from build123d import *

# Parameters (mm, degrees)
SKETCH1_W           = 164.45
SKETCH1_H           = 80
SKETCH1_R           = 2.5
SKETCH1_W_2         = 43.25
SKETCH1_H_2         = 50
BOSS_EXTRUDE1_DEPTH = 3.1
SKETCH2_W           = 3.1
SKETCH2_H           = 39.596362368
SKETCH2_H_2         = 40
CUT_EXTRUDE1_DEPTH  = 4.1
FILLET1_R           = 25
SKETCH3_R           = 2.5
BOSS_EXTRUDE2_DEPTH = 3.1
FILLET3_R           = 10
FILLET4_R           = 20


with BuildPart() as part:
    # Sketch1 → Boss-Extrude1 (new body)
    with BuildSketch(Plane.XY):
        Rectangle(SKETCH1_W, SKETCH1_H)
        Circle(SKETCH1_R, mode=Mode.SUBTRACT)
        with BuildLine():
            Line((-76.75, -15.97), (-76.75, 15.97))
            ThreePointArc((-76.75, 15.97), (-75, 17.72), (-73.25, 15.97))
            Line((-73.25, 15.97), (-73.25, -15.97))
            ThreePointArc((-73.25, -15.97), (-75, -17.72), (-76.75, -15.97))
        make_face(mode=Mode.SUBTRACT)
        with BuildLine():
            Line((18.725, -15.97), (18.725, 15.97))
            ThreePointArc((18.725, 15.97), (20.475, 17.72), (22.225, 15.97))
            Line((22.225, 15.97), (22.225, -15.97))
            ThreePointArc((22.225, -15.97), (20.475, -17.72), (18.725, -15.97))
        make_face(mode=Mode.SUBTRACT)
        with Locations((-36.625, 0)):
            Rectangle(SKETCH1_W_2, SKETCH1_H_2, mode=Mode.SUBTRACT)
    extrude(amount=BOSS_EXTRUDE1_DEPTH)

    # Sketch2 → Cut-Extrude1 (cut, through all)
    with BuildSketch(Plane.XY.offset(3.1)):
        with Locations((61.575, -20.201818816)):
            Rectangle(SKETCH2_W, SKETCH2_H)
        with Locations((80.675, -20)):
            Rectangle(SKETCH2_W, SKETCH2_H_2)
    extrude(amount=-CUT_EXTRUDE1_DEPTH, mode=Mode.SUBTRACT)

    # Fillet1
    fillet1_edges = [part.edges().sort_by_distance(p)[0] for p in [
        (-82.225, -40, 1.55),
        (-82.225, 40, 1.55),
    ]]
    fillet(fillet1_edges, radius=FILLET1_R)

    # Sketch3 → Boss-Extrude2 (add)
    with BuildSketch(Plane.XY.offset(3.1)):
        with BuildLine():
            add(Edge.make_bspline(
                [(82.225, 40), (100.790922155, 40.44036534), (122.998075296, 29.670027282), (145.632337886, 10.163727788), (160, 10)],
                knots=[0, 0, 0, 0, 0.531248583, 1, 1, 1, 1], degree=3))
            Line((82.225, 40), (82.225, -40))
            add(Edge.make_bspline(
                [(82.225, -40), (100.790922155, -40.44036534), (122.998075296, -29.670027282), (145.632337886, -10.163727788), (160, -10)],
                knots=[0, 0, 0, 0, 0.531248583, 1, 1, 1, 1], degree=3))
            Line((160, -10), (160, 10))
        make_face()
        with Locations((150, 0)):
            Circle(SKETCH3_R, mode=Mode.SUBTRACT)
    extrude(amount=-BOSS_EXTRUDE2_DEPTH)

    # Fillet3
    fillet3_edges = [part.edges().sort_by_distance(p)[0] for p in [
        (160, -10, 1.55),
        (160, 10, 1.55),
    ]]
    fillet(fillet3_edges, radius=FILLET3_R)

    # Fillet4
    fillet4_edges = [part.edges().sort_by_distance(p)[0] for p in [
        (-15, -25, 1.55),
        (-15, 25, 1.55),
        (-58.25, 25, 1.55),
        (-58.25, -25, 1.55),
    ]]
    fillet(fillet4_edges, radius=FILLET4_R)


solid = part.part
The listing builds one solid part. Answer for the finished solid, in the listing's coordinates (mm). A direction names the side the tool comes from. Give positions to 0.01 mm unless a question says otherwise; leave off trailing zeros. Write each loop counter-clockwise with the first axis right and the second up, starting at its lowest first coordinate (ties: lowest second). Pieces come first, ordered by that corner, then holes.
Item 1: Section B-B, the plane z = 1.5 is taken. Count the separate pieces of the cut face and the enclosed holes in it, plus the area to 3 significant figures.
Item 2: Flat-ended cylindrical pins translate along their axes: P1, Ø1.6, axis at y = -27.5, z = 1.5, coming from the +X side; P2, Ø1.5, axis at x = 76, z = 0.5, coming from the +Y side; P3, Ø1.5, axis at x = 75, z = 2, coming from the -Y side. Find the tip coordinate at first contact, or state that the pin passes through.
Item 3: Which of the six approach directions +Z, -Z, +X, -X, +Y, -Y give full straight-line access (tool end or side, diameter ignored) to faces 1 (the flat face through (41, 1, 3.1)), 2 (the cylindrical face through (-20.703, 18.986, 1.572))?
Item 4: Determine the mould class of faces 3 (the flat face through (41, 1, 0)), 4 (the cylindrical face through (152.385, 0.751, 1.572)), 5 (the cylindrical face through (-75.1, -32.48, 1.57)), 6 (the cylindrical face through (-21.014, -19.297, 1.572)) for opening direction X: released by +X, released by -X, zero draft, split by the parting line, or undercut.
Item 5: Find the intervals of material crossed by line 1 along Y through (x, z) = (0, 0.95); line 2 along X through (y, z) = (1, 0.9) (3 decimals); line 3 along X through (y, z) = (-3, 1.45) (3 decimals), in increasing order.
Item 6: Section A-A, the plane x = 0 is taken. Write down the section's boundary in (y, z).
Completed:
1. separate pieces: 1
1. enclosed holes: 5
1. area: 14,700 mm2
2. P1: stops at x = 124.26
2. P2: stops at y = 40
2. P3: stops at y = -40
3. face 1: +Z, +X, -X, +Y, -Y
3. face 2: +Z, -Z
4. face 3: zero draft
4. face 4: undercut
4. face 5: released by -X
4. face 6: undercut
5. line 1: y = -40 to -2.5, 2.5 to 40
5. line 2: x = -82.225 to -76.75, -73.25 to -58.25, -15 to -2.291, 2.291 to 18.725, 22.225 to 147.709, 152.291 to 160
5. line 3: x = -82.225 to -76.75, -73.25 to -58.25, -15 to 18.725, 22.225 to 60.025, 63.125 to 79.125, 82.225 to 159.843
6. outline: (-40, 0) - (-2.5, 0) - (-2.5, 3.1) - (-40, 3.1) - close; (2.5, 0) - (40, 0) - (40, 3.1) - (2.5, 3.1) - close
